The drawing under review shows one solid part. Ordinate dimensions are in mm from its lowest x, y, z. Coordinates: 2 decimals unless noted, no trailing zeros. Loops run counter-clockwise (first coordinate to the right, second up) from the corner with the lowest first, then second, coordinate; pieces in that order, holes last. Notation, with made-up numbers: M -14.5,70.25 L 13.5,70.25 A17 cw 13.5,93.25 Z; hole C -6,-28.75 d1. An arc over 180 degrees is marked long. Return JSON: item names as keys, results as strings.
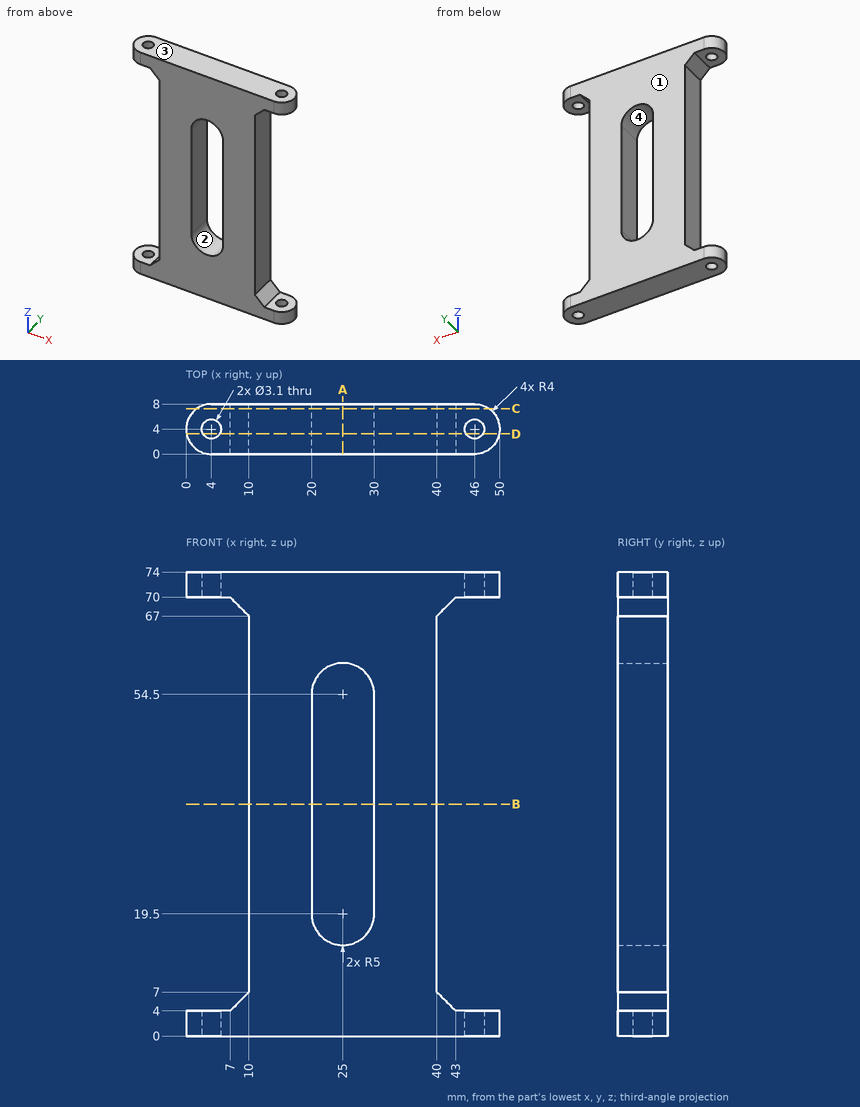
1. To check wall thickness, follow line 1 (Y direction, x = 4, z = 71); line 2 (Z direction, x = 44, y = 7.25); line 3 (X direction, y = 7, z = 34). State the ranges of each line that lie inside material, in increasing order.
Check values:
{"line 1": "0 to 2.45, 5.55 to 8", "line 2": "0 to 4, 70 to 74", "line 3": "10 to 20, 30 to 40"}
2. Add section B-B on z = 37. Give the boundary of the cut face in (x, y).
Check values:
{"outline": "M 10,0 L 20,0 L 20,8 L 10,8 Z; M 30,0 L 40,0 L 40,8 L 30,8 Z"}
3. The part is to be moulded in two halves that separate along Z. For the marked faces 1, 2, 3 and 4, say which applies: released by +Z, released by -Z, zero draft, split by the parting line, or undercut.
Check values:
{"face 1": "zero draft", "face 2": "undercut", "face 3": "released by +Z", "face 4": "undercut"}
4. Add section D-D on y = 3.25. State how many separate pieces and enclosed holes the cut face has, plus the area to 4 significant figures.
Check values:
{"separate pieces": "5", "enclosed holes": "1", "area": "1,925 mm²"}
5. Add section A-A on x = 25. Give the boundary of the cut face in (y, z).
Check values:
{"outline": "M 0,0 L 8,0 L 8,14.5 L 0,14.5 Z; M 0,59.5 L 8,59.5 L 8,74 L 0,74 Z"}
6. Add section C-C on y = 7.25. Give the boundary of the cut face in (x, z), plus the area to 3 significant figures.
Check values:
{"outline": "M 1.67,0 L 48.33,0 L 48.33,4 L 43,4 L 40,7 L 40,67 L 43,70 L 48.33,70 L 48.33,74 L 1.67,74 L 1.67,70 L 7,70 L 10,67 L 10,7 L 7,4 L 1.67,4 Z; hole M 20,19.5 A5 ccw 30,19.5 L 30,54.5 A5 ccw 20,54.5 Z", "area": "1,940 mm²"}
7. Insertion check: pin 1 Ø1.5 at (y, z) = (3.5, 55) entering from -X; pin 2 Ø1 at (y, z) = (7, 53) entering from +X; pin 3 Ø3 at (x, y) = (4, 4) entering from +Z. Each pin has a flat end and moves straight along its axis. Give the tip position at first contact, or say it passes through.
Check values:
{"pin 1": "x = 10", "pin 2": "x = 40", "pin 3": "through"}
